Input: part model. Units: mm. Frame: model coordinates. A direction names the side the tool comes from. Round coordinates to 2 decimals unless told otherwise and drop trailing zeros. Write each loop counter-clockwise with the first axis right and the second up, starting at its lowest first coordinate (ties: lowest second). Pieces come first, ordered by that corner, then holes. Notation, with made-up numbers: (57.25, -14) - (94.25, -14) arc R24 ccw to (94.25, 7) - close; hole circle Ø3 at (-0.75, -33). An arc over 180 degrees is marked (long way). One line per item, written item: value. Start each with the question number.
```python
from build123d import *

# Parameters (mm, degrees)
BOSS_EXTRUDE1_DEPTH     = 7.8
SKETCH2_R               = 3.6
BOSS_EXTRUDE2_DEPTH     = 2.2
BOSS_EXTRUDE3_START     = 0.4
SKETCH3_R               = 3.6
BOSS_EXTRUDE3_DEPTH     = 0.4
CUT_EXTRUDE1_DEPTH      = 13.583057392
CUT_EXTRUDE1_DEPTH_BACK = 13.583057392
SKETCH4_R               = 2.5


with BuildPart() as part:
    # Sketch1 → Boss-Extrude1 (new body)
    with BuildSketch(Plane(origin=(0, 0, 0), x_dir=(1, 0, 0), z_dir=(0, 1, 0))):
        Polygon((5.773502692, 0), (2.886751346, 5), (-2.886751346, 5), (-5.773502692, 0), (-2.886751346, -5), (2.886751346, -5), align=None)
    extrude(amount=BOSS_EXTRUDE1_DEPTH)

    # Sketch2 → Boss-Extrude2 (add)
    with BuildSketch(Plane(origin=(0, 7.8, 0), x_dir=(1, 0, 0), z_dir=(0, 1, 0))):
        with Locations(Location((0, 0, 0), (0, 0, 270))):
            Circle(SKETCH2_R)
    extrude(amount=BOSS_EXTRUDE2_DEPTH)

    # Sketch3 → Boss-Extrude3 (add)
    with BuildSketch(Plane.XZ.offset(BOSS_EXTRUDE3_START)):
        with Locations(Location((0, 0, 0), (0, 0, 90))):
            Circle(SKETCH3_R)
    extrude(amount=-BOSS_EXTRUDE3_DEPTH)

    # Sketch4 → Cut-Extrude1 (cut, two sides: drawn at the far end of the back side and taken through both)
    with BuildSketch(Plane(origin=(0, 0, 0), x_dir=(1, 0, 0), z_dir=(0, 1, 0)).offset(-CUT_EXTRUDE1_DEPTH_BACK)):
        with Locations(Location((0.8, 0, 0), (0, 0, 270))):
            Circle(SKETCH4_R)
    extrude(amount=CUT_EXTRUDE1_DEPTH + CUT_EXTRUDE1_DEPTH_BACK, mode=Mode.SUBTRACT)


solid = part.part
```
Q1. Cut plane A-A, the plane y = 7. Output: boundary loops of the cut face in (x, z), and give its area (3 significant figures).
Q2. Material intervals for probe 1 along Z at (x, y) = (0.8, 7); probe 2 along Y at (x, z) = (-2, 4); probe 3 along Z at (x, y) = (2.75, 6.5), sorted ascending. Write a range as from..to.
Q3. Pull-direction query (Z, two-part tool) for faces 1 (the flat face through (-4.31, 3.845, -2.535)), 2 (the flat face through (-2, -0.4, 1)), 3 (the flat face through (-4.35, 3.845, 2.465)), 4 (the cylindrical face through (1.551, 4.727, 2.385)); classes: pulls with the +Z half, pulls with the -Z half, needs draft (parallel to the pull), parting line crosses it, or undercut.
Q4. Cut plane B-B, the plane x = 1.5. Output: boundary loops of the cut face in (y, z).
Q5. Contact query for flat-ended pins moving along their axis: pin 1 Ø5 at (y, z) = (2.5, -1) entering from +X; pin 2 Ø4 at (y, z) = (8.5, -2.5) entering from +X; pin 3 Ø5 at (y, z) = (4.5, -1) entering from -X. Output: stop coordinate, or through.
Q6. Cut plane C-C, the plane x = -2.25. Output: boundary loops of the cut face in (y, z).
Q7. Access query for faces 5 (the cylindrical face through (1.379, -0.203, 3.325)), 6 (the flat face through (4.31, 3.845, 2.535)), 7 (the flat face through (4, 7.8, 0)). Directions: +Z, -Z, +X, -X, +Y, -Y. A direction counts if a zero-diameter tool reaches every point of the face in a straight line with its end or side. Return the directions, or none.
Q8. Cut plane D-D, the plane x = 0. Output: boundary loops of the cut face in (y, z), and give its area (3 significant figures).
A:
1. outline: (-5.77, 0) - (-2.89, -5) - (2.89, -5) - (5.77, 0) - (2.89, 5) - (-2.89, 5) - close; hole circle Ø5 at (0.8, 0)
1. area: 67.0 mm²
2. probe 1: z = -5..-2.5, 2.5..5
2. probe 2: y = 0..7.8
2. probe 3: z = -5..-1.56, 1.56..5
3. face 1: pulls with the -Z half
3. face 2: needs draft
3. face 3: pulls with the +Z half
3. face 4: undercut
4. outline: (-0.4, -3.27) - (0, -3.27) - (0, -5) - (7.8, -5) - (7.8, -3.27) - (10, -3.27) - (10, -2.4) - (-0.4, -2.4) - close; (-0.4, 2.4) - (10, 2.4) - (10, 3.27) - (7.8, 3.27) - (7.8, 5) - (0, 5) - (0, 3.27) - (-0.4, 3.27) - close
5. pin 1: stops at x = 5.77
5. pin 2: stops at x = 5.41
5. pin 3: stops at x = -5.77
6. outline: (-0.4, -2.81) - (0, -2.81) - (0, -5) - (7.8, -5) - (7.8, -2.81) - (10, -2.81) - (10, 2.81) - (7.8, 2.81) - (7.8, 5) - (0, 5) - (0, 2.81) - (-0.4, 2.81) - close
7. face 5: -Y
7. face 6: +Z, +X, +Y, -Y
7. face 7: +Y
8. outline: (-0.4, -3.6) - (0, -3.6) - (0, -5) - (7.8, -5) - (7.8, -3.6) - (10, -3.6) - (10, -2.37) - (-0.4, -2.37) - close; (-0.4, 2.37) - (10, 2.37) - (10, 3.6) - (7.8, 3.6) - (7.8, 5) - (0, 5) - (0, 3.6) - (-0.4, 3.6) - close
8. area: 47.5 mm²
